Here's how the part is built. I have some questions about the finished solid (model axes, mm). Face numbers are marked on the shaded views. A direction names the side the tool comes from. Coordinates: 2 decimals unless noted, no trailing zeros. Loops run counter-clockwise (first coordinate to the right, second up) from the corner with the lowest first, then second, coordinate; pieces in that order, holes last. Notation, with made-up numbers: (0, 50.5) - (53, 50.5) arc R22 ccw to (53, 88.5) - close; hole circle Ø2 at (4.25, 38.5). An arc over 180 degrees is marked (long way). Use a Markdown table: item, result.
```python
from build123d import *

# Parameters (mm, degrees)
F0_R     = 203.2
F0_W     = 812.8
F0_H     = 457.2
F1_DEPTH = 1016
F2_W     = 634.4814898748
F2_H     = 454.6432495117
F3_DEPTH = 812.801
F4_W     = 457.2
F4_H     = 279.4
F5_DEPTH = 812.8
F7_DEPTH = 812.8


with BuildPart() as f1:
    # F0 (on Top) → F1 (new body)
    with BuildSketch(Plane.XY):
        with BuildLine():
            Line((589.4354466658, 298.5482140541), (-324.9645533342, 298.5482140541))
            ThreePointArc((-324.9645533342, 298.5482140541), (-731.3645533342, -107.8517859459), (-324.9645533342, -514.2517859459))
            Line((-324.9645533342, -514.2517859459), (589.4354466658, -514.2517859459))
            Line((589.4354466658, -514.2517859459), (589.4354466658, -336.4517859459))
            Line((589.4354466658, -336.4517859459), (589.4354466658, 120.7482140541))
            Line((589.4354466658, 120.7482140541), (589.4354466658, 298.5482140541))
        make_face()
        with Locations((-324.9645533342, -107.8517859459)):
            Circle(F0_R, mode=Mode.SUBTRACT)
        with Locations((995.8354466658, -107.8517859459)):
            Rectangle(F0_W, F0_H)
    extrude(amount=F1_DEPTH)

    # F2 (on face) → F3 (cut, through all)
    with BuildSketch(Plane(origin=(0, 298.5482140541, 0), x_dir=(-1, 0, 0), z_dir=(0, 1, 0))):
        with Locations((7.7238083968, 509.9283456802)):
            Rectangle(F2_W, F2_H)
        Polygon((324.9645533342, 737.2499704361), (324.9645533342, 282.6067209244), (821.0112452507, 282.6067209244), (892.6659226418, 737.2499704361), align=None)
    extrude(amount=-F3_DEPTH, mode=Mode.SUBTRACT)

    # F4 (on face) → F5 (cut)
    with BuildSketch(Plane.YZ.offset(1402.2354466658)):
        with Locations((-107.8517859459, 876.3)):
            Rectangle(F4_W, F4_H)
        with Locations((-107.8517859459, 139.7)):
            Rectangle(F4_W, F4_H)
    extrude(amount=-F5_DEPTH, mode=Mode.SUBTRACT)

    # F6 (on face) → F7 (cut)
    with BuildSketch(Plane.YZ.offset(1402.2354466658)):
        with BuildLine():
            Line((120.7482140541, 736.6), (-107.8517859459, 736.6))
            ThreePointArc((-107.8517859459, 736.6), (53.7928242334, 669.6446101792), (120.7482140541, 508))
            Line((120.7482140541, 508), (120.7482140541, 736.6))
        make_face()
        with BuildLine():
            ThreePointArc((120.7482140541, 508), (53.7928242333, 346.3553898207), (-107.8517859459, 279.4))
            Line((-107.8517859459, 279.4), (120.7482140541, 279.4))
            Line((120.7482140541, 279.4), (120.7482140541, 508))
        make_face()
        with BuildLine():
            Line((-336.4517859459, 508), (-336.4517859459, 279.4))
            Line((-336.4517859459, 279.4), (-107.8517859459, 279.4))
            ThreePointArc((-107.8517859459, 279.4), (-269.4963961252, 346.3553898208), (-336.4517859459, 508))
        make_face()
        with BuildLine():
            Line((-336.4517859459, 736.6), (-336.4517859459, 508))
            ThreePointArc((-336.4517859459, 508), (-269.4963961251, 669.6446101792), (-107.8517859459, 736.6))
            Line((-107.8517859459, 736.6), (-336.4517859459, 736.6))
        make_face()
    extrude(amount=-F7_DEPTH, mode=Mode.SUBTRACT)


solid = f1.part
```
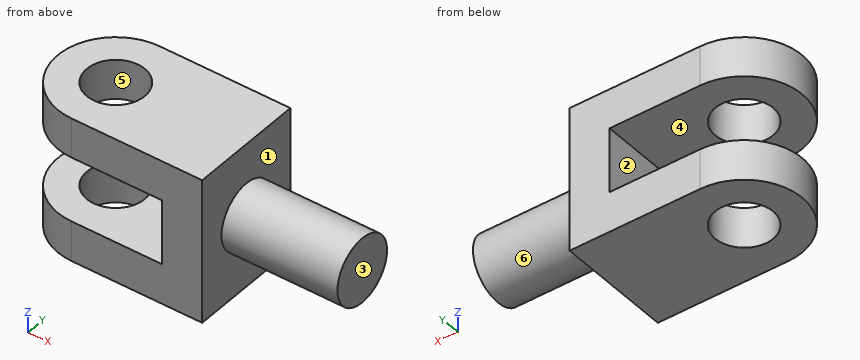
Q1. I want a section at C-C, the plane y = 26.5. Write out the boundary of the cut face in (x, z), then the cut area to 3 significant figures.
Check values:
| item | result |
|---|---|
| outline | (-708.51, 0) - (-477.41, 0) - (-477.41, 282.61) - (-708.51, 282.61) - close; (-708.51, 737.25) - (-477.41, 737.25) - (-477.41, 1016) - (-708.51, 1016) - close; (-172.52, 0) - (589.44, 0) - (589.44, 323.05) - (1402.24, 323.05) - (1402.24, 692.95) - (589.44, 692.95) - (589.44, 1016) - (-172.52, 1016) - (-172.52, 737.25) - (309.52, 737.25) - (309.52, 282.61) - (-172.52, 282.61) - close |
| area | 985,000 mm^2 |
Q2. Will these pins go through, and if not, where does the flat tip stop? P1, Ø4, axis at y = -259.5, z = 489, coming from the -X side; P2, Ø12, axis at y = 193, z = 877, coming from the -X side; P3, Ø4, axis at y = 9, z = 796, coming from the -X side; P4, Ø5, axis at x = 397, y = -172.5, coming from the -Z side.
Check values:
| item | result |
|---|---|
| P1 | x = 309.52 |
| P2 | x = -604.65 |
| P3 | x = -714.8 |
| P4 | z = 0 |
Q3. I want a section at D-D, the plane y = -396. Write out the boundary of the cut face in (x, z), then the cut area to 3 significant figures.
Check values:
| item | result |
|---|---|
| outline | (-611.55, 0) - (589.44, 0) - (589.44, 1016) - (-611.55, 1016) - (-611.55, 737.25) - (309.52, 737.25) - (309.52, 282.61) - (-611.55, 282.61) - close |
| area | 801,000 mm^2 |
Q4. Please list where these lines run through material, in increasing order: L1, parallel to Z at x = 4.5, y = 238.5; L2, parallel to X at y = -36.5, z = 188.5; L3, parallel to X at y = -433.5, z = 662. Write a range as from..to.
Check values:
| item | result |
|---|---|
| L1 | 0..282.61, 737.25..1016 |
| L2 | -725.05..-515.23, -134.7..589.44 |
| L3 | 309.52..589.44 |
Q5. If we mould it in two halves opening along Y, with no side actions, what happens to the marked faces 4, 5 and 6? For each: pulls with the +Y half, pulls with the -Y half, needs draft (parallel to the pull), parting line crosses it, or undercut.
Check values:
| item | result |
|---|---|
| face 4 | needs draft |
| face 5 | undercut |
| face 6 | parting line crosses it |
Q6. I want a section at A-A, the plane x = -58.5. Write out the boundary of the cut face in (y, z), then the cut area to 3 significant figures.
Check values:
| item | result |
|---|---|
| outline | (-514.25, 0) - (298.55, 0) - (298.55, 282.61) - (-514.25, 282.61) - close; (-514.25, 737.25) - (298.55, 737.25) - (298.55, 1016) - (-514.25, 1016) - close |
| area | 456,000 mm^2 |
Q7. I want a section at B-B, the plane z = 508. Write out the boundary of the cut face in (x, y), then the cut area to 3 significant figures.
Check values:
| item | result |
|---|---|
| outline | (309.52, -514.25) - (589.44, -514.25) - (589.44, -336.45) - (1402.24, -336.45) - (1402.24, 120.75) - (589.44, 120.75) - (589.44, 298.55) - (309.52, 298.55) - close |
| area | 599,000 mm^2 |
Q8. Which directions (+Z, -Z, +X, -X, +Y, -Y) give clear straight access to the entire face, cutting with the end or side of a thin tool? Please do the marked faces 1, 2 and 3.
Check values:
| item | result |
|---|---|
| face 1 | +X |
| face 2 | -X, +Y, -Y |
| face 3 | +Z, -Z, +X, +Y, -Y |
